```python
from build123d import *

# Parameters (mm, degrees)
SKETCH_1_W          = 40
SKETCH_1_H          = 39
EXTRUDE_1_DEPTH     = 20
SKETCH_3_R          = 6
EXTRUDE_2_DEPTH     = 1
SKETCH_4_R          = 3
EXTRUDE_4_DEPTH     = 25.5
SKETCH_5_W          = 20
SKETCH_5_H          = 1.515151515
EXTRUDE_5_DEPTH     = 8
SKETCH_6_W          = 19.988535735
SKETCH_6_H          = 1.420485619
EXTRUDE_8_DEPTH     = 8
SKETCH_7_R          = 1.710468594
SKETCH_7_R_2        = 1.604618823
SKETCH_7_R_3        = 2
CUT_EXTRUDE_2_DEPTH = 3
SKETCH_9_R          = 5.273794996
EXTRUDE_9_DEPTH     = 1.5


with BuildPart() as part:
    # 草图1 → 凸台-拉伸1 (new body)
    with BuildSketch(Plane.XY):
        Rectangle(SKETCH_1_W, SKETCH_1_H)
    extrude(amount=EXTRUDE_1_DEPTH)

    # 草图3 → 凸台-拉伸2 (add)
    with BuildSketch(Plane(origin=(0, 19.5, 0), x_dir=(1, 0, 0), z_dir=(0, 1, 0))):
        with Locations(Location((-10, -10, 0), (0, 0, 90))):
            Circle(SKETCH_3_R)
    extrude(amount=EXTRUDE_2_DEPTH)

    # 草图4 → 凸台-拉伸4 (add)
    with BuildSketch(Plane(origin=(0, 0, 0), x_dir=(1, 0, 0), z_dir=(0, 1, 0))):
        with Locations(Location((-10, -10, 0), (0, 0, 270))):
            Circle(SKETCH_4_R)
    extrude(amount=EXTRUDE_4_DEPTH)

    # 草图5 → 凸台-拉伸5 (add)
    with BuildSketch(Plane.ZY.offset(20)):
        with Locations((10, 7.757575758)):
            Rectangle(SKETCH_5_W, SKETCH_5_H)
    extrude(amount=EXTRUDE_5_DEPTH)

    # 草图6 → 凸台-拉伸8 (add)
    with BuildSketch(Plane(origin=(20, 0, 0), x_dir=(0, 0, -1), z_dir=(1, 0, 0))):
        with Locations((-9.994267868, 7.493661874)):
            Rectangle(SKETCH_6_W, SKETCH_6_H)
    extrude(amount=EXTRUDE_8_DEPTH)

    # 草图7 → 切除-拉伸2 (cut)
    with BuildSketch(Plane(origin=(0, 8.515151515, 0), x_dir=(1, 0, 0), z_dir=(0, 1, 0))):
        with Locations(Location((-24, -5, 0), (0, 0, 270))):
            Circle(SKETCH_7_R)
        with Locations(Location((-24, -15, 0), (0, 0, 270))):
            Circle(SKETCH_7_R_2)
        with Locations(Location((23.963224728, -5, 0), (0, 0, 270))):
            Circle(SKETCH_7_R_3)
        with Locations(Location((23.963224728, -15, 0), (0, 0, 270))):
            Circle(SKETCH_7_R_3)
    extrude(amount=-CUT_EXTRUDE_2_DEPTH, mode=Mode.SUBTRACT)

    # 草图9 → 凸台-拉伸9 (add)
    with BuildSketch(Plane(origin=(0, 19.5, 0), x_dir=(1, 0, 0), z_dir=(0, 1, 0))):
        with Locations(Location((-10, -10, 0), (0, 0, 270))):
            Circle(SKETCH_9_R)
    extrude(amount=EXTRUDE_9_DEPTH)


solid = part.part
```
The listing builds one solid part. Answer for the finished solid, in the listing's coordinates (mm). A direction names the side the tool comes from. Coordinates: 2 decimals unless noted, no trailing zeros. Write each loop counter-clockwise with the first axis right and the second up, starting at its lowest first coordinate (ties: lowest second). Pieces come first, ordered by that corner, then holes.
Q1. Section A-A, the plane x = -24 is taken. Write down the section's boundary in (y, z), then the cut area to 3 significant figures.
Returned:
outline: (7, 0) - (8.52, 0) - (8.52, 3.29) - (7, 3.29) - close; (7, 6.71) - (8.52, 6.71) - (8.52, 13.4) - (7, 13.4) - close; (7, 16.6) - (8.52, 16.6) - (8.52, 20) - (7, 20) - close
area: 20.3 mm2
Q2. Find the intervals of material crossed by line 1 along X through (y, z) = (7.9, 15); line 2 along X through (y, z) = (7.85, 5); line 3 along X through (y, z) = (13.5, 16.75), in increasing order.
Returned:
line 1: x = -28 to -25.6, -22.4 to 21.96, 25.96 to 28
line 2: x = -28 to -25.71, -22.29 to 21.96, 25.96 to 28
line 3: x = -20 to 20
Q3. Section B-B, the plane z = 10 is taken. Write down the section's boundary in (x, y).
Returned:
outline: (-28, 7) - (-20, 7) - (-20, -19.5) - (20, -19.5) - (20, 6.78) - (28, 6.78) - (28, 8.2) - (20, 8.2) - (20, 19.5) - (-4, 19.5) - (-4, 20.5) - (-4.73, 20.5) - (-4.73, 21) - (-7, 21) - (-7, 25.5) - (-13, 25.5) - (-13, 21) - (-15.27, 21) - (-15.27, 20.5) - (-16, 20.5) - (-16, 19.5) - (-20, 19.5) - (-20, 8.52) - (-28, 8.52) - close
Q4. Section D-D, the plane y = 2 is taken. Write down the section's boundary in (x, z), then the cut area to 3 significant figures.
Returned:
outline: (-20, 0) - (20, 0) - (20, 20) - (-20, 20) - close
area: 800 mm2
Q5. Given P1, Ø6, axis at y = -7, z = 8, coming from the +X side; P2, Ø2.5, axis at x = 22.5, z = 15, coming from the +Y side; P3, Ø1.1, axis at x = 24, y = 7.5, coming from the +Z side, each flat-ended and moving along its own axis, determine where each tip first touches the part or whether it passes through.
Returned:
P1: stops at x = 20
P2: stops at y = 8.2
P3: stops at z = 19.99
Q6. Which of the six approach directions +Z, -Z, +X, -X, +Y, -Y give full straight-line access (tool end or side, diameter ignored) to faces 5 (the flat face through (-24, 8.515, 10)), 6 (the flat face through (-20, -6, 10)), 7 (the flat face through (24, 8.204, 10)), 8 (the flat face through (20, 0, 10)), 9 (the flat face through (-6, 20.5, 6))?
Returned:
face 5: +Z, -Z, -X, +Y
face 6: +Z, -Z, -X, -Y
face 7: +Z, -Z, +X, +Y
face 8: +Z, -Z, +X
face 9: +Y
Q7. The mould has two halves that part along Z. Classify faces 1 (the flat face through (-20, 14, 10)), 2 (the flat face through (24, 7, 19.989)), 3 (the cylindrical face through (24, 8, 3)), 4 (the cylindrical face through (-4.677, 19.993, 7.231)): released by +Z, released by -Z, zero draft, split by the parting line, or undercut.
Returned:
face 1: zero draft
face 2: released by +Z
face 3: undercut
face 4: split by the parting line
Q8. Section C-C, the plane x = -11.5 is taken. Write down the section's boundary in (y, z).
Returned:
outline: (-19.5, 0) - (19.5, 0) - (19.5, 4.19) - (20.5, 4.19) - (20.5, 4.94) - (21, 4.94) - (21, 7.4) - (25.5, 7.4) - (25.5, 12.6) - (21, 12.6) - (21, 15.06) - (20.5, 15.06) - (20.5, 15.81) - (19.5, 15.81) - (19.5, 20) - (-19.5, 20) - close
